Check sheet for the drawn part. Datum: minimum x, y, z corner. Units: mm. A direction names the side the tool comes from. Coordinates: 2 decimals unless noted, no trailing zeros. Order: outer loops, then holes, each group sorted by start corner. A loop starts at its lowest first (then second) coordinate and runs counter-clockwise, first axis right, second up. Notation, with made-up numbers: (-2, 10.25) - (3, 10.25) arc R28 ccw to (3, 35.25) - close; hole circle Ø8 at (-33.5, -3). An arc over 180 degrees is marked (long way). Put each result on its own line as item: value.
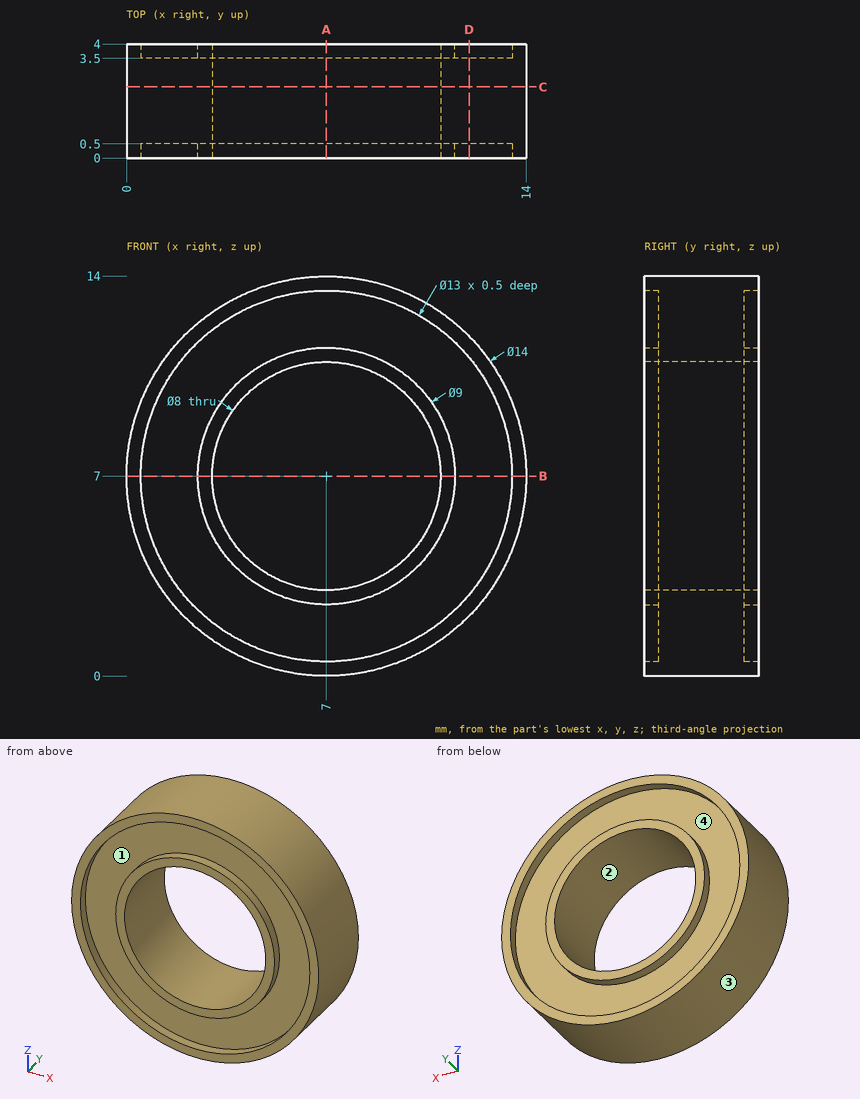
Q1. Section check D-D on x = 12. Record the boundary of the cut face in (y, z).
Answer block:
outline: (0, 2.1) - (4, 2.1) - (4, 2.85) - (3.5, 2.85) - (3.5, 11.15) - (4, 11.15) - (4, 11.9) - (0, 11.9) - (0, 11.15) - (0.5, 11.15) - (0.5, 2.85) - (0, 2.85) - close
Q2. Section check B-B on z = 7. Record the boundary of the cut face in (x, y), then the cut area to 3 significant figures.
Answer block:
outline: (0, 0) - (0.5, 0) - (0.5, 0.5) - (2.5, 0.5) - (2.5, 0) - (3, 0) - (3, 4) - (2.5, 4) - (2.5, 3.5) - (0.5, 3.5) - (0.5, 4) - (0, 4) - close; (11, 0) - (11.5, 0) - (11.5, 0.5) - (13.5, 0.5) - (13.5, 0) - (14, 0) - (14, 4) - (13.5, 4) - (13.5, 3.5) - (11.5, 3.5) - (11.5, 4) - (11, 4) - close
area: 20.0 mm^2
Q3. Depth check by flat-ended pin: pin 1 Ø4 at (x, z) = (9, 9.5) entering from -Y. Enter the tip coordinate at first touch or a pass-through.
Answer block:
pin 1: stops at y = 0
Q4. Draft check along Z on the marked faces 3 and 4. Enter one of: pulls with the +Z half, pulls with the -Z half, needs draft (parallel to the pull), parting line crosses it, or undercut.
Answer block:
face 3: parting line crosses it
face 4: undercut
Q5. Thickness scan on L1, parallel to Z at x = 7, y = 3.6; L2, parallel to Z at x = 7, y = 1.7. Record the ranges inside material, lowest first. Write a range as [from, to].
Answer block:
L1: z = [0, 0.5], [2.5, 3], [11, 11.5], [13.5, 14]
L2: z = [0, 3], [11, 14]
Q6. Section check A-A on x = 7. Record the boundary of the cut face in (y, z), then the cut area to 3 significant figures.
Answer block:
outline: (0, 0) - (4, 0) - (4, 0.5) - (3.5, 0.5) - (3.5, 2.5) - (4, 2.5) - (4, 3) - (0, 3) - (0, 2.5) - (0.5, 2.5) - (0.5, 0.5) - (0, 0.5) - close; (0, 11) - (4, 11) - (4, 11.5) - (3.5, 11.5) - (3.5, 13.5) - (4, 13.5) - (4, 14) - (0, 14) - (0, 13.5) - (0.5, 13.5) - (0.5, 11.5) - (0, 11.5) - close
area: 20.0 mm^2
Q7. Section check C-C on y = 2.5. Record the boundary of the cut face in (x, z), then the cut area to 3 significant figures.
Answer block:
outline: circle Ø14 at (7, 7); hole circle Ø8 at (7, 7)
area: 104 mm^2
Q8. Access from +Z, -Z, +X, -X, +Y, -Y to the whole of each face (thin tool, end or side, straight path). Record for the marked faces 1 and 2.
Answer block:
face 1: -Y
face 2: +Y, -Y
